Autodesk Inventor part; units mm, degrees
ref_plane "YZ Plane" through (0, 0, 0) normal (1, 0, 0) x (0, 1, 0)
ref_plane "XZ Plane" through (0, 0, 0) normal (0, 1, 0) x (-1, 0, 0)
ref_plane "XY Plane" through (0, 0, 0) normal (0, 0, 1) x (1, 0, 0)
sketch "Sketch1" plane through (0, 0, 0) normal (0, 0, 1) x (1, 0, 0)
  line L0 (-12.7, 25.4) -> (12.7, 25.4)
  line L1 (12.7, 25.4) -> (12.7, -25.4)
  line L2 (12.7, -25.4) -> (-12.7, -25.4)
  line L3 (-12.7, -25.4) -> (-12.7, 25.4)
  line L4 (9.525, 22.225) -> (-9.525, 22.225)
  line L5 (-9.525, 22.225) -> (-9.525, -22.225)
  line L6 (-9.525, -22.225) -> (9.525, -22.225)
  line L7 (9.525, -22.225) -> (9.525, 22.225)
  point P0 (0, 0)
  point P1 (0, 0)
  point P2 (0, 25.4)
  point P3 (-12.7, 0)
extrude "Extrusion1" add sketch "Sketch1" along normal blind 457.2
properties part number "Aluminum Box Tube" material "Aluminum 6061"
Geometry: final body of the model. Coordinates: model frame, mm. A direction names the side the tool comes from. Round coordinates to 2 decimals unless told otherwise and drop trailing zeros. Order: outer loops, then holes, each group sorted by start corner. A loop starts at its lowest first (then second) coordinate and runs counter-clockwise, first axis right, second up. Notation, with made-up numbers: (-12.5, 66.5) -> (-2.5, 66.5) arc R18 cw to (-2.5, 80.5) -> close; hole circle Ø10 at (13.5, 47). An arc over 180 degrees is marked (long way). Use one line per item in the form item = value. Start each with the question number.
1. Cut plane B-B (z = 59.5). Return the cut outline in (x, y) (3 decimals), then the cut area to 3 significant figures.
2. Cut plane C-C (y = 13). Return the cut outline in (x, z) (3 decimals), then the cut area to 3 significant figures.
3. Cut plane A-A (x = 5). Return the cut outline in (y, z) (3 decimals), then the cut area to 3 significant figures.
4. Reachability of faces 1 (the face through (-9.525, 0, 225)), 2 (the face through (-12.7, 0, 225)) from +Z, -Z, +X, -X, +Y, -Y: full face, straight path, thin tool, end or side. Return the list, or none.
5. Draft query along Y for faces 3 (the face through (0, -25.4, 225)), 4 (the face through (12.7, 0, 225)), 5 (the face through (0, 22.225, 225)). Return one class per face: pulls with the +Y half, pulls with the -Y half, needs draft (parallel to the pull), parting line crosses it, or undercut.
6. Line query: probe 1 along Y at (x, z) = (5, 68) (3 decimals); probe 2 along X at (y, z) = (18, 327) (3 decimals). Output: solid intervals per line, ascending.
Solution:
q1.outline = (-12.7, -25.4) -> (12.7, -25.4) -> (12.7, 25.4) -> (-12.7, 25.4) -> close; hole (-9.525, -22.225) -> (9.525, -22.225) -> (9.525, 22.225) -> (-9.525, 22.225) -> close
q1.area = 444 mm^2
q2.outline = (-12.7, 0) -> (-9.525, 0) -> (-9.525, 457.2) -> (-12.7, 457.2) -> close; (9.525, 0) -> (12.7, 0) -> (12.7, 457.2) -> (9.525, 457.2) -> close
q2.area = 2,900 mm^2
q3.outline = (-25.4, 0) -> (-22.225, 0) -> (-22.225, 457.2) -> (-25.4, 457.2) -> close; (22.225, 0) -> (25.4, 0) -> (25.4, 457.2) -> (22.225, 457.2) -> close
q3.area = 2,900 mm^2
q4.face_1 = +Z, -Z
q4.face_2 = +Z, -Z, -X, +Y, -Y
q5.face_3 = pulls with the -Y half
q5.face_4 = needs draft
q5.face_5 = undercut
q6.probe_1 = -25.4 to -22.225, 22.225 to 25.4
q6.probe_2 = -12.7 to -9.525, 9.525 to 12.7
